Geometry check sheet. Reference: the model listing, model coordinates, mm. A direction names the side the tool comes from. Give positions to 0.01 mm unless a question says otherwise; leave off trailing zeros. Write each loop counter-clockwise with the first axis right and the second up, starting at its lowest first coordinate (ties: lowest second). Pieces come first, ordered by that corner, then holes. Notation, with made-up numbers: (-3, 74) - (49, 74) arc R23 cw to (49, 82) - close; hole circle Ø6 at (81.5, 51.25). An arc over 180 degrees is marked (long way). One line per question, with ' | ' between items. Start each with the question number.
Q1. Thickness scan on L1, parallel to X at y = 14, z = 11; L2, parallel to Z at x = 27, y = -6.5 (3 decimals). Record the ranges inside material, lowest first. Write a range as [from, to].
Q2. Section check B-B on y = 5. Record the boundary of the cut face in (x, z) (3 decimals), and give its area (3 significant figures).
Q3. Section check A-A on z = -29. Record the boundary of the cut face in (x, y).
Q4. Set-up check for faces 1 (the face through (41.57, -1, 1)), 2 (the face through (-43, -1, 38.1)): record each of +Z, -Z, +X, -X, +Y, -Y from which the full face is reachable in a straight line by a thin tool's end or side.
Q5. Section check C-C on x = 27. Record the boundary of the cut face in (y, z) (3 decimals).
Q6. Gauge pin test, flat end, axial feed: P1, Ø4, axis at x = -6.5, y = 31, coming from the +Z side (3 decimals). Record the tip position at first contact, or that the pin passes through.
```python
from build123d import *

# Parameters (mm, degrees)
F0_W     = 88.9
F0_H     = 76.2
F1_DEPTH = 44.45
F2_W     = 82.55
F2_H     = 73.025
F3_DEPTH = 44.45


with BuildPart() as f1:
    # F0 (on Front) → F1 (new body, symmetric)
    with BuildSketch(Plane.XZ):
        Rectangle(F0_W, F0_H)
    extrude(amount=F1_DEPTH, both=True)

    # F2 (on Front) → F3 (cut, symmetric)
    with BuildSketch(Plane.XZ):
        with Locations((0.2950895578, 1.5875)):
            Rectangle(F2_W, F2_H)
    extrude(amount=F3_DEPTH, both=True, mode=Mode.SUBTRACT)


solid = f1.part
```
Working result:
1) L1: x = [-44.45, -40.98], [41.57, 44.45] | L2: z = [-38.1, -34.925]
2) outline: (-44.45, -38.1) - (44.45, -38.1) - (44.45, 38.1) - (41.57, 38.1) - (41.57, -34.925) - (-40.98, -34.925) - (-40.98, 38.1) - (-44.45, 38.1) - close | area: 746 mm2
3) outline: (-44.45, -44.45) - (-40.98, -44.45) - (-40.98, 44.45) - (-44.45, 44.45) - close; (41.57, -44.45) - (44.45, -44.45) - (44.45, 44.45) - (41.57, 44.45) - close
4) face 1: +Z, +Y, -Y | face 2: +Z, +X, -X, +Y, -Y
5) outline: (-44.45, -38.1) - (44.45, -38.1) - (44.45, -34.925) - (-44.45, -34.925) - close
6) P1: stops at z = -34.925
